The model under review builds one solid part; all positions refer to its coordinate system, in mm. Face numbers are marked on the shaded views. A direction names the side the tool comes from. Coordinates: 2 decimals unless noted, no trailing zeros. Order: outer loops, then holes, each group sorted by start corner. A loop starts at its lowest first (then second) coordinate and runs counter-clockwise, first axis right, second up.
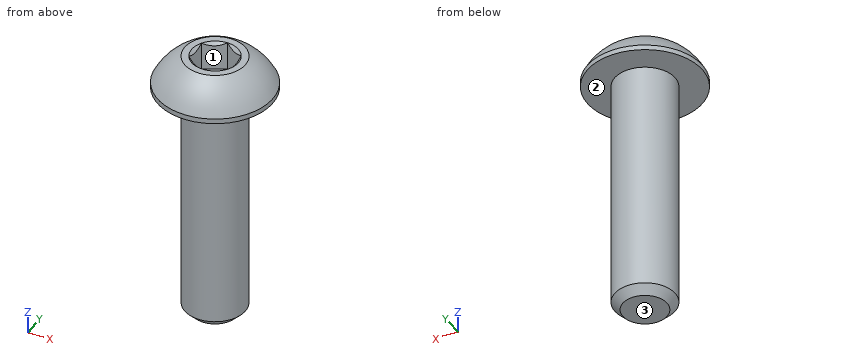
```python
from build123d import *

# Parameters (mm, degrees)
CUT_EXTRUDE1_DEPTH = 1.4


with BuildPart() as part:
    # Sketch2 → Revolve1 (revolve)
    with BuildSketch(Plane(origin=(0, 0, 0), x_dir=(0, 0, -1), z_dir=(1, 0, 0)), mode=Mode.PRIVATE) as revolve1_sk:
        with BuildLine():
            Line((-6.825, 0), (6.825, 0))
            Line((6.825, 0), (6.825, 1.1))
            Line((6.825, 1.1), (6.425, 1.5))
            Line((6.425, 1.5), (-5.175, 1.5))
            Line((-5.175, 1.5), (-5.175, 2.85))
            Line((-5.175, 2.85), (-5.4225, 2.85))
            ThreePointArc((-5.4225, 2.85), (-6.22987489, 2.285251969), (-6.825, 1.5))
            Line((-6.825, 1.5), (-6.825, 0))
        make_face()
    revolve(revolve1_sk.sketch.rotate(Axis((0, 0, 6.825), (0, 0, -1)), 90), axis=Axis((0, 0, 6.825), (0, 0, -1)))

    # Sketch3 → Cut-Extrude1 (cut)
    with BuildSketch(Plane.XY.offset(6.825)):
        Polygon((0, 1.154700538), (-1, 0.577350269), (-1, -0.577350269), (0, -1.154700538), (1, -0.577350269), (1, 0.577350269), align=None)
    extrude(amount=-CUT_EXTRUDE1_DEPTH, mode=Mode.SUBTRACT)

    # Cut-Extrude2 cone 1 section (through the dimple's axis) → Cut-Extrude2 (revolve, cut)
    with BuildSketch(Plane(origin=(0, 0, 6.825), x_dir=(0, -1, 0), z_dir=(1, 0, 0))):
        Polygon((0, 0), (1.154700538, 0), (0, 1.154700538), align=None)
    revolve(axis=Axis((0, 0, 6.825), (0, 0, -1)), mode=Mode.SUBTRACT)


solid = part.part
```
(1) Wall thickness on probe 1 along Y at (x, z) = (-1.7, 6.25); probe 2 along X at (y, z) = (-1, 6.25): over which ranges is each line inside the solid? List them lowest first.
A:
probe 1: y = -1.5 to 1.5
probe 2: x = -2.03 to -0.27, 0.27 to 2.03
(2) We need section B-B, the plane z = 6. Write out the cut boundary in (x, y).
A:
outline: circle Ø4.97 at (0, 0); hole (-1, -0.58) - (0, -1.15) - (1, -0.58) - (1, 0.58) - (0, 1.15) - (-1, 0.58) - close
(3) Machinability: for the marked faces 1, 2 and 3, which of the approach directions +Z, -Z, +X, -X, +Y, -Y give a long, thin tool a straight path to every point of the face, cutting with its end or side? Answer none if there is none.
A:
face 1: +Z
face 2: -Z
face 3: -Z, +X, -X, +Y, -Y
(4) For pin 1 Ø2 at (y, z) = (0.5, -2.5) entering from +X; pin 2 Ø3 at (x, z) = (0, -2) entering from +Y; pin 3 Ø2 at (x, y) = (-0.5, 0.5) entering from +Z (3 decimals); pin 4 Ø0.6 at (y, z) = (0, 6.5) entering from +X, all flat-tipped, find the tip position at first contact; note any pin that passes through.
A:
pin 1: stops at x = 1.5
pin 2: stops at y = 1.5
pin 3: stops at z = 6.825
pin 4: stops at x = 2.31
(5) We need section C-C, the plane z = 3.25. Write out the cut boundary in (x, y).
A:
outline: circle Ø3 at (0, 0)
